Autodesk Inventor part; units mm, degrees
ref_plane "YZ Plane" through (0, 0, 0) normal (1, 0, 0) x (0, 1, 0)
ref_plane "XZ Plane" through (0, 0, 0) normal (0, 1, 0) x (-1, 0, 0)
ref_plane "XY Plane" through (0, 0, 0) normal (0, 0, 1) x (1, 0, 0)
sketch "Sketch1" plane through (0, 0, 0) normal (0, 1, 0) x (-1, 0, 0)
  line L0 (-17.75, -17.75) -> (17.75, -17.75)
  line L1 (17.75, -17.75) -> (17.75, 17.75)
  line L2 (17.75, 17.75) -> (-17.75, 17.75)
  line L3 (-17.75, 17.75) -> (-17.75, -17.75)
  line L4 (-17.75, -17.75) -> (17.75, 17.75) construction
  line L5 (17.75, -17.75) -> (-17.75, 17.75) construction
  line L6 (-2.45, -12.65) -> (2.45, -12.65) construction
  line L7 (2.45, -12.65) -> (2.45, 12.65) construction
  line L8 (2.45, 12.65) -> (-2.45, 12.65) construction
  line L9 (-2.45, 12.65) -> (-2.45, -12.65) construction
  line L10 (-2.45, -12.65) -> (2.45, 12.65) construction
  line L11 (2.45, -12.65) -> (-2.45, 12.65) construction
  line L12 (-12.65, -2.45) -> (12.65, -2.45) construction
  line L13 (12.65, -2.45) -> (12.65, 2.45) construction
  line L14 (12.65, 2.45) -> (-12.65, 2.45) construction
  line L15 (-12.65, 2.45) -> (-12.65, -2.45) construction
  line L16 (-12.65, -2.45) -> (12.65, 2.45) construction
  line L17 (12.65, -2.45) -> (-12.65, 2.45) construction
  line L18 (-12.85, -2.65) -> (12.85, -2.65)
  line L19 (12.85, -2.65) -> (12.85, 2.65)
  line L20 (12.85, 2.65) -> (-12.85, 2.65)
  line L21 (-12.85, 2.65) -> (-12.85, -2.65)
  line L22 (-12.85, -2.65) -> (12.85, 2.65) construction
  line L23 (12.85, -2.65) -> (-12.85, 2.65) construction
  line L24 (-2.65, -12.85) -> (2.65, -12.85)
  line L25 (2.65, -12.85) -> (2.65, 12.85)
  line L26 (2.65, 12.85) -> (-2.65, 12.85)
  line L27 (-2.65, 12.85) -> (-2.65, -12.85)
  line L28 (-2.65, -12.85) -> (2.65, 12.85) construction
  line L29 (2.65, -12.85) -> (-2.65, 12.85) construction
  point P0 (0, 0)
  point P1 (0, 0)
  dimension "d0" = 35.5
  dimension "d1" = 4.9
  dimension "d2" = 10.2
  dimension "d3" = 0.2
  dimension "d4" = 0.2
extrude "Extrusion1" add sketch "Sketch1" along normal blind 1.9
sketch "Sketch2" plane through (0, 1.9, 0) normal (0, 1, 0) x (1, 0, 0)
  line L0 (17.75, 17.75) -> (-17.75, 17.75)
  line L1 (-17.75, 17.75) -> (-17.75, -17.75)
  line L2 (-17.75, -17.75) -> (17.75, -17.75)
  line L3 (17.75, -17.75) -> (17.75, 17.75)
  circle A0 centre (0, 0) radius 1.5
  dimension "d7" = 3
extrude "Extrusion2" add sketch "Sketch2" along normal blind 2
sketch "Sketch3" plane through (0, 3.9, 0) normal (0, 1, 0) x (1, 0, 0)
  circle A0 centre (0, 0) radius 1.5
  line L0 (17.75, 17.75) -> (-17.75, 17.75)
  line L1 (-17.75, 17.75) -> (-17.75, -17.75)
  line L2 (-17.75, -17.75) -> (17.75, -17.75)
  line L3 (17.75, -17.75) -> (17.75, 17.75)
  circle A1 centre (0, 0) radius 2.75
  dimension "d10" = 5.5
extrude "Extrusion3" add sketch "Sketch3" along normal blind 2.5 contours L3 L2 L1 L0
chamfer "Chamfer1" distance 2 angle 45 1 edges at (-2.65, 0.95, -2.65)
fillet "Fillet1" radius 2.45 1 edges at (-12.85, 0.95, -2.65)
fillet "Fillet2" radius 2.45 1 edges at (-2.65, 0.95, -12.85)
chamfer "Chamfer2" distance 2 angle 45 1 edges at (2.65, 0.95, -2.65)
chamfer "Chamfer3" distance 2 angle 45 1 edges at (2.65, 0.95, 2.65)
fillet "Fillet3" radius 2.45 1 edges at (12.85, 0.95, -2.65)
fillet "Fillet4" radius 2.45 1 edges at (2.65, 0.95, -12.85)
fillet "Fillet5" radius 2.45 1 edges at (12.85, 0.95, 2.65)
fillet "Fillet6" radius 2.45 1 edges at (2.65, 0.95, 12.85)
chamfer "Chamfer4" distance 2 angle 45 1 edges at (-2.65, 0.95, 2.65)
fillet "Fillet7" radius 2.45 2 edges at (-2.65, 0.95, 12.85) (-12.85, 0.95, 2.65)
equation "\"d0\" = 3 * ServoArmLength + ServoArmWidth"
equation "\"d1\" = ServoArmWidth"
equation "\"d2\" = ServoArmLength"
equation "\"d3\" = ServoArmSpacing"
equation "\"d4\" = ServoArmSpacing"
equation "\"d5\" = ServoArmThickness"
equation "\"d7\" = ServoArmHoleRequired"
equation "\"d8\" = MinimalThickness"
equation "\"d10\" = ServoArmHeadScrewTrace"
equation "\"d11\" = ServoArmHeadScrewThickness"
equation "\"d13\" = ServoArmInternFillet"
equation "\"d16\" = ServoArmExternFillet"
equation "\"d17\" = ServoArmExternFillet"
equation "\"d18\" = ServoArmInternFillet"
equation "\"d21\" = ServoArmInternFillet"
equation "\"d24\" = ServoArmExternFillet"
equation "\"d25\" = ServoArmExternFillet"
equation "\"d26\" = ServoArmExternFillet"
equation "\"d27\" = ServoArmExternFillet"
equation "\"d28\" = ServoArmInternFillet"
equation "\"d31\" = ServoArmExternFillet"
properties part number "CoronaArmTrace"
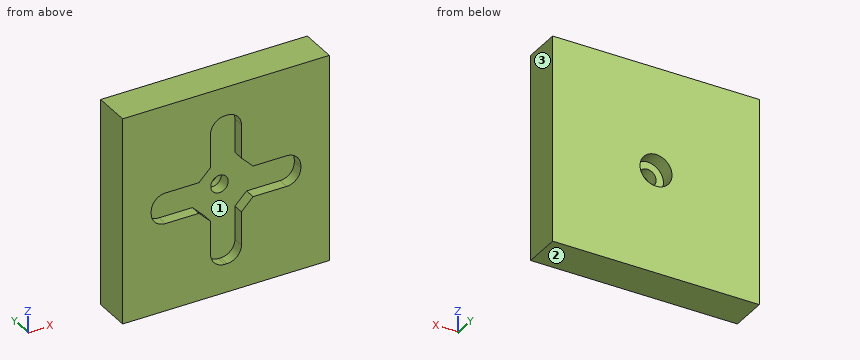
Input: part model. Units: mm. Frame: model coordinates. Face numbers are marked on the shaded views. Give positions to 0.01 mm unless a question says otherwise; leave off trailing zeros. Loops run counter-clockwise (first coordinate to the right, second up) from the corner with the lowest first, then second, coordinate; pieces in that order, holes last. Notation, with made-up numbers: M 72,60 L 109,60 A21 ccw 109,97 Z; hole C 49,45.25 d2. An arc over 180 degrees is marked long. Use CSV: the item, a comma, the result in double quotes.
(1) Section B-B, the plane x = -8. Return loops of the section in (y, z), plus the area to 3 significant figures.
Outcome:
outline,"M 0,-17.75 L 6.4,-17.75 L 6.4,17.75 L 0,17.75 L 0,2.65 L 1.9,2.65 L 1.9,-2.65 L 0,-2.65 Z"
area,"217 mm²"
(2) Section C-C, the plane z = -4. Return loops of the section in (x, y).
Outcome:
outline,"M -17.75,0 L -3.3,0 L -3.3,1.9 L 3.3,1.9 L 3.3,0 L 17.75,0 L 17.75,6.4 L -17.75,6.4 Z"
(3) Material intervals for L1, parallel to X at y = 2.55, z = 0; L2, parallel to X at y = 5.5, z = 0, sorted ascending. Write a range as [from, to].
Outcome:
L1,"x = [-17.75, -1.5], [1.5, 17.75]"
L2,"x = [-17.75, -2.75], [2.75, 17.75]"
(4) Section A-A, the plane y = 1. Return loops of the section in (x, z), plus the area to 3 significant figures.
Outcome:
outline,"M -17.75,-17.75 L 17.75,-17.75 L 17.75,17.75 L -17.75,17.75 Z; hole M -12.85,-0.2 A2.45 ccw -10.4,-2.65 L -4.65,-2.65 L -2.65,-4.65 L -2.65,-10.4 A2.45 ccw -0.2,-12.85 L 0.2,-12.85 A2.45 ccw 2.65,-10.4 L 2.65,-4.65 L 4.65,-2.65 L 10.4,-2.65 A2.45 ccw 12.85,-0.2 L 12.85,0.2 A2.45 ccw 10.4,2.65 L 4.65,2.65 L 2.65,4.65 L 2.65,10.4 A2.45 ccw 0.2,12.85 L -0.2,12.85 A2.45 ccw -2.65,10.4 L -2.65,4.65 L -4.65,2.65 L -10.4,2.65 A2.45 ccw -12.85,0.2 Z"
area,"1,020 mm²"
(5) Pull-direction query (Z, two-part tool) for the marked faces 1, 2 and 3; classes: pulls with the +Z half, pulls with the -Z half, needs draft (parallel to the pull), parting line crosses it, or undercut.
Outcome:
face 1,"undercut"
face 2,"pulls with the -Z half"
face 3,"needs draft"
(6) Section D-D, the plane y = 5. Return loops of the section in (x, z), plus the area to 3 significant figures.
Outcome:
outline,"M -17.75,-17.75 L 17.75,-17.75 L 17.75,17.75 L -17.75,17.75 Z; hole C 0,0 d5.5"
area,"1,240 mm²"
(7) Pin query (flat end, axial travel): P1, Ø4, axis at x = 11.5, z = -13.5, coming from the -Y side; P2, Ø5, axis at x = 0, z = 0, coming from the +Y side. Return the tip coordinate at first contact, or that it passes through.
Outcome:
P1,"stops at y = 0"
P2,"stops at y = 3.9"
